Check sheet for the modelled part. Datum: model origin and axes. Units: mm. Face numbers are marked on the shaded views. Coordinates: 2 decimals unless noted, no trailing zeros. Loops run counter-clockwise (first coordinate to the right, second up) from the corner with the lowest first, then second, coordinate; pieces in that order, holes last. Notation, with made-up numbers: M 18,44.25 L 52,44.25 A8 cw 52,59.25 Z; hole C 69.5,16 d1. An arc over 180 degrees is marked long. Return JSON: item names as keys, results as strings.
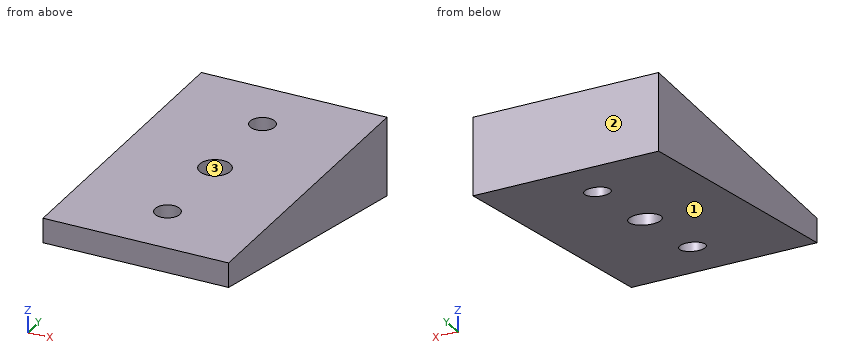
from build123d import *

# Parameters (mm, degrees)
BOSS_EXTRUDE1_DEPTH = 30
SKETCH3_R           = 4
SKETCH3_R_2         = 5
CUT_EXTRUDE1_DEPTH  = 60


with BuildPart() as part:
    # Sketch2 → Boss-Extrude1 (new, symmetric)
    with BuildSketch(Plane(origin=(0, 0, 0), x_dir=(0, 0, -1), z_dir=(1, 0, 0))):
        Polygon((4, 50), (21.632698071, 50), (4, -50), (-4, -50), (-4, 50), align=None)
    extrude(amount=BOSS_EXTRUDE1_DEPTH, both=True)

    # Sketch3 → Cut-Extrude1 (cut)
    with BuildSketch(Plane.XY.offset(4)):
        with Locations((0, -30)):
            Circle(SKETCH3_R)
        with Locations((0, 30)):
            Circle(SKETCH3_R)
        Circle(SKETCH3_R_2)
    extrude(amount=-CUT_EXTRUDE1_DEPTH, mode=Mode.SUBTRACT)


solid = part.part
1) Section check C-C on x = 0. Record the cut outline in (y, z), then the cut area to 3 significant figures.
Answers:
{"outline": "M -50,-4 L -34,-6.82 L -34,4 L -50,4 Z; M -26,-8.23 L -5,-11.93 L -5,4 L -26,4 Z; M 5,-13.7 L 26,-17.4 L 26,4 L 5,4 Z; M 34,-18.81 L 50,-21.63 L 50,4 L 34,4 Z", "area": "1,240 mm²"}
2) Draft check along Y on the marked faces 1, 2 and 3. Enter one of: +Y half, -Y half, draft (parallel to the pull), parting line (faces both ways), or undercut.
Answers:
{"face 1": "-Y half", "face 2": "+Y half", "face 3": "undercut"}
3) Section check A-A on z = 0. Record the cut outline in (x, y).
Answers:
{"outline": "M -30,-50 L 30,-50 L 30,50 L -30,50 Z; hole C 0,0 d10; hole C 0,-30 d8; hole C 0,30 d8"}
4) Section check D-D on y = -30. Record the cut outline in (x, z), then the cut area to 3 significant figures.
Answers:
{"outline": "M -30,-7.53 L -4,-7.53 L -4,4 L -30,4 Z; M 4,-7.53 L 30,-7.53 L 30,4 L 4,4 Z", "area": "599 mm²"}
5) Scan lines: line 1 along Y through (x, z) = (0, 1.5); line 2 along X through (y, z) = (-30, 0.75); line 3 along Y through (x, z) = (1, -3.25). Record each from-to range of solid material in increasing order. Write a range as [from, to].
Answers:
{"line 1": "[-50, -34], [-26, -5], [5, 26], [34, 50]", "line 2": "[-30, -4], [4, 30]", "line 3": "[-50, -33.87], [-26.13, -4.9], [4.9, 26.13], [33.87, 50]"}
6) Section check B-B on y = 0. Record the cut outline in (x, z), then the cut area to 3 significant figures.
Answers:
{"outline": "M -30,-12.82 L -5,-12.82 L -5,4 L -30,4 Z; M 5,-12.82 L 30,-12.82 L 30,4 L 5,4 Z", "area": "841 mm²"}
7) Go/stop test with flat-tipped pins: pin 1 Ø5 at (x, y) = (-21.5, -26.5) entering from -Z; pin 2 Ø1.5 at (x, y) = (-21, -22) entering from -Z. Record where each tip stops, or that it passes through.
Answers:
{"pin 1": "z = -8.58", "pin 2": "z = -9.07"}
